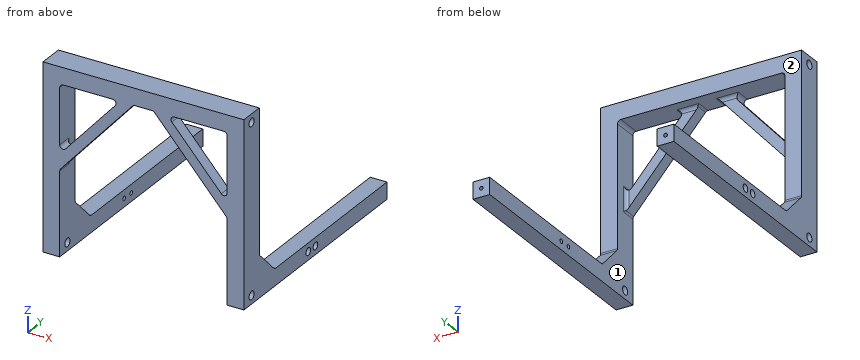
from build123d import *

# Parameters (mm, degrees)
BOSS_EXTRUDE1_DEPTH   = 19.05
SKETCH2_W             = 12.7
SKETCH2_H             = 158.75
BOSS_EXTRUDE2_DEPTH   = 12.7
BOSS_EXTRUDE2_2_DEPTH = 12.7
BOSS_EXTRUDE3_DEPTH   = 12.7
BOSS_EXTRUDE4_DEPTH   = 12.7
SKETCH5_R             = 1.5875
CUT_EXTRUDE1_DEPTH    = 273.680564031
SKETCH6_R             = 2.8575
CUT_EXTRUDE2_DEPTH    = 5.08
BOSS_EXTRUDE5_DEPTH   = 8.89
SKETCH8_R             = 1.397
CUT_EXTRUDE3_DEPTH    = 12.7
FILLET1_R             = 2.54
SKETCH9_R             = 3.175
CUT_EXTRUDE4_DEPTH    = 273.680564031


with BuildPart() as part:
    # Sketch1 → Boss-Extrude1 (new body)
    with BuildSketch(Plane(origin=(0, 0, 0), x_dir=(1, 0, 0), z_dir=(0, 1, 0))):
        Polygon((-76.2, 139.7), (-76.2, 0), (76.2, 0), (76.2, 139.7), (63.5, 139.7), (63.5, 12.7), (-63.5, 12.7), (-63.5, 139.7), align=None)
    extrude(amount=BOSS_EXTRUDE1_DEPTH)



with BuildPart() as body_2:
    # Sketch2 → Boss-Extrude2 (new body)
    with BuildSketch(Plane(origin=(0, 0, -139.7), x_dir=(-1, 0, 0), z_dir=(0, 0, -1))):
        with Locations((-69.85, 98.425)):
            Rectangle(SKETCH2_W, SKETCH2_H)
    extrude(amount=-BOSS_EXTRUDE2_DEPTH)


with BuildPart() as body_3:
    # Sketch2 → Boss-Extrude2 2 (new body)
    with BuildSketch(Plane(origin=(0, 0, -139.7), x_dir=(-1, 0, 0), z_dir=(0, 0, -1))):
        with Locations((69.85, 98.425)):
            Rectangle(SKETCH2_W, SKETCH2_H)
    extrude(amount=-BOSS_EXTRUDE2_2_DEPTH)


with BuildPart() as part_1:
    add(part.part)

    add(body_2.part)  # Boss-Extrude3 merges body 2
    # Sketch3 → Boss-Extrude3 (add)
    with BuildSketch(Plane(origin=(76.2, 0, 0), x_dir=(0, 0, -1), z_dir=(1, 0, 0))):
        Polygon((127, 38.1), (107.95, 19.05), (127, 19.05), align=None)
    extrude(amount=-BOSS_EXTRUDE3_DEPTH)


    add(body_3.part)  # Boss-Extrude4 merges body 3
    # Sketch4 → Boss-Extrude4 (add)
    with BuildSketch(Plane.ZY.offset(76.2)):
        Polygon((-127, 38.1), (-107.95, 19.05), (-127, 19.05), align=None)
    extrude(amount=-BOSS_EXTRUDE4_DEPTH)

    # Sketch5 → Cut-Extrude1 (cut, through all)
    with BuildSketch(Plane(origin=(76.2, 0, 0), x_dir=(0, 0, -1), z_dir=(1, 0, 0))):
        with Locations((133.35, 88.9)):
            Circle(SKETCH5_R)
        with Locations((133.35, 80.01)):
            Circle(SKETCH5_R)
    extrude(amount=-CUT_EXTRUDE1_DEPTH, mode=Mode.SUBTRACT)

    # Sketch6 → Cut-Extrude2 (cut)
    with BuildSketch(Plane(origin=(76.2, 0, 0), x_dir=(0, 0, -1), z_dir=(1, 0, 0))):
        with Locations((133.35, 88.9)):
            Circle(SKETCH6_R)
        with Locations(Location((133.35, 80.01, 0), (0, 0, 180))):
            Circle(SKETCH6_R)
    cut_extrude2 = extrude(amount=-CUT_EXTRUDE2_DEPTH, mode=Mode.SUBTRACT)

    # Mirror2: Cut-Extrude2 across plane
    add(cut_extrude2.mirror(Plane(origin=(0, 0, 0), x_dir=(0, 0, 1), z_dir=(1, 0, 0))), mode=Mode.SUBTRACT)

    # Sketch7 → Boss-Extrude5 (add)
    with BuildSketch(Plane.XZ):
        Polygon((-17.797608372, -12.7), (-63.5, -64.115190582), (-63.5, -75.584809418), (-7.602391628, -12.7), align=None)
        Polygon((7.602391628, -12.7), (17.797608372, -12.7), (63.5, -64.115190582), (63.5, -75.584809418), align=None)
    extrude(amount=-BOSS_EXTRUDE5_DEPTH)

    # Sketch8 → Cut-Extrude3 (cut)
    with BuildSketch(Plane(origin=(0, 177.8, 0), x_dir=(1, 0, 0), z_dir=(0, 1, 0))):
        with Locations(Location((69.85, 133.35, 0), (0, 0, 270))):
            Circle(SKETCH8_R)
    cut_extrude3 = extrude(amount=-CUT_EXTRUDE3_DEPTH, mode=Mode.SUBTRACT)

    # Mirror3: Cut-Extrude3 across plane
    add(cut_extrude3.mirror(Plane(origin=(0, 0, 0), x_dir=(0, 0, 1), z_dir=(1, 0, 0))), mode=Mode.SUBTRACT)

    # Fillet1
    fillet1_edges = [part_1.edges().sort_by_distance(p)[0] for p in [
        (63.5, 4.445, -75.584809418),
        (12.7, 8.89, -12.7),
        (7.602391628, 4.445, -12.7),
        (17.797608372, 4.445, -12.7),
        (63.5, 8.89, -69.85),
        (63.5, 4.445, -64.115190582),
        (-69.85, 19.05, -107.95),
        (-69.85, 38.1, -127),
        (63.5, 9.525, -12.7),
        (-63.5, 9.525, -12.7),
        (69.85, 19.05, -107.95),
        (69.85, 38.1, -127),
        (-12.7, 8.89, -12.7),
        (-17.797608372, 4.445, -12.7),
        (-7.602391628, 4.445, -12.7),
        (-63.5, 8.89, -69.85),
        (-63.5, 4.445, -75.584809418),
        (-63.5, 4.445, -64.115190582),
    ]]
    fillet(fillet1_edges, radius=FILLET1_R)

    # Sketch9 → Cut-Extrude4 (cut, through all)
    with BuildSketch(Plane(origin=(76.2, 0, 0), x_dir=(0, 0, -1), z_dir=(1, 0, 0))):
        with Locations((6.35, 9.525)):
            Circle(SKETCH9_R)
        with Locations((133.35, 9.525)):
            Circle(SKETCH9_R)
    extrude(amount=-CUT_EXTRUDE4_DEPTH, mode=Mode.SUBTRACT)


solid = part_1.part
Design review of the part built by this model. Coordinates are the model's own, in mm. Face numbers are marked on the shaded views. Round coordinates to 2 decimals unless told otherwise and drop trailing zeros. Write each loop counter-clockwise with the first axis right and the second up, starting at its lowest first coordinate (ties: lowest second). Pieces come first, ordered by that corner, then holes. Notation, with made-up numbers: (59, 18.5) -> (78, 18.5) arc R19 ccw to (78, 44.5) -> close; hole circle Ø11 at (88.25, 46.5). An arc over 180 degrees is marked (long way). One line per item, written item: value. Start each with the question number.
Q1. Insertion check: P1, Ø4, axis at y = 80.01, z = -133.35, coming from the +X side; P2, Ø10, axis at x = 59.5, y = 111.5, coming from the +Z side; P3, Ø5, axis at y = 9.525, z = -6.35, coming from the -X side; P4, Ø5, axis at y = 88.9, z = -133.35, coming from the -X side. Each pin has a flat end and moves straight along its axis. Give the tip position at first contact, or say it passes through.
Q2. Add section B-B (y = 35). Give the boundary of the cut face in (x, z), then the cut area to 3 significant figures.
Q3. Add section A-A (z = -86.5). Give the boundary of the cut face in (x, y), then the cut area to 3 significant figures.
Q4. Add section C-C (x = 56). Give the boundary of the cut face in (y, z) (3 decimals).
Q5. To check wall thickness, follow probe 1 along Y at (x, z) = (-72.55, -133.35); probe 2 along X at (y, z) = (18.5, -89.5); probe 3 along Z at (x, y) = (72.5, 80.01). State the ranges of each line that lie inside material, in increasing order.
Q6. Add section D-D (z = -19.5). Give the boundary of the cut face in (x, y).
Q7. The part is to be moulded in two halves that separate along Z. For the marked faces 1 and 2, say which applies: pulls with the +Z half, pulls with the -Z half, needs draft (parallel to the pull), parting line crosses it, or undercut.
Response:
1. P1: stops at x = 71.12
1. P2: stops at z = -127
1. P3: passes through
1. P4: stops at x = -71.12
2. outline: (-76.2, -139.7) -> (-63.5, -139.7) -> (-63.5, -123.9) -> (-76.2, -123.9) -> close; (63.5, -139.7) -> (76.2, -139.7) -> (76.2, -123.9) -> (63.5, -123.9) -> close
2. area: 401 mm^2
3. outline: (-76.2, 0) -> (-63.5, 0) -> (-63.5, 19.05) -> (-76.2, 19.05) -> close; (63.5, 0) -> (76.2, 0) -> (76.2, 19.05) -> (63.5, 19.05) -> close
3. area: 484 mm^2
4. outline: (0, -67.147) -> (8.89, -67.147) -> (8.89, -55.678) -> (0, -55.678) -> close; (0, -12.7) -> (19.05, -12.7) -> (19.05, 0) -> (0, 0) -> close; hole circle Ø6.35 at (9.525, -6.35)
5. probe 1: y = 0 to 6.35, 12.7 to 77.15, 82.87 to 86.04, 91.76 to 177.8
5. probe 2: x = -76.2 to -63.5, 63.5 to 76.2
5. probe 3: z = -139.7 to -136.21, -130.49 to -127
6. outline: (-76.2, 0) -> (-63.5, 0) -> (-63.5, 19.05) -> (-76.2, 19.05) -> close; (-23.84, 0) -> (-13.65, 0) -> (-13.65, 8.89) -> (-23.84, 8.89) -> close; (13.65, 0) -> (23.84, 0) -> (23.84, 8.89) -> (13.65, 8.89) -> close; (63.5, 0) -> (76.2, 0) -> (76.2, 19.05) -> (63.5, 19.05) -> close
7. face 1: undercut
7. face 2: needs draft
